Build history of the part. All positions in model axes, mm. Round coordinates to 2 decimals unless told otherwise and drop trailing zeros. Write each loop counter-clockwise with the first axis right and the second up, starting at its lowest first coordinate (ties: lowest second). Pieces come first, ordered by that corner, then holes.
1) Wall check: probe 1 along Y at (x, z) = (-49.5, 1.35); probe 2 along X at (y, z) = (5.5, -0.4); probe 3 along X at (y, z) = (3.75, -1.1). Give the ranges that are in metal, low to high.
2) Saw through at C-C (x = 53). Write the cut outline in (y, z).
3) Saw through at B-B (y = 0). Write the cut outline in (x, z).
4) Saw through at A-A (z = -0.05). Write the cut outline in (x, y).
5) Saw through at D-D (y = -10). Write the cut outline in (x, z).
6) Flat gauge pins, fed straight in: pin 1 (1 mm diameter, centred on y = 9.5, z = -0.5, fed in from -X); pin 2 (1 mm diameter, centred on y = 9, z = 0.5, fed in from -X); pin 3 (1 mm diameter, centred on y = -2, z = -1, fed in from +X). Where does each tip first touch, or does it go through?
Autodesk Inventor part; units mm, degrees
ref_plane "YZ Plane" through (0, 0, 0) normal (1, 0, 0) x (0, 1, 0)
ref_plane "XZ Plane" through (0, 0, 0) normal (0, 1, 0) x (-1, 0, 0)
ref_plane "XY Plane" through (0, 0, 0) normal (0, 0, 1) x (1, 0, 0)
sketch "Esboço1" plane through (0, 0, 0) normal (0, 0, 1) x (1, 0, 0)
  line L0 (-49.5, 0) -> (49.5, 0) construction
  line L1 (-49.5, -15) -> (49.5, -15)
  line L2 (49.5, 15) -> (-49.5, 15)
  arc A0 (-49.5, 15) -> (-49.5, -15) centre (-49.5, 0) ccw
  arc A1 (49.5, -15) -> (49.5, 15) centre (49.5, 0) ccw
  circle A2 centre (-49.5, 0) radius 8
  circle A3 centre (49.5, 0) radius 8
  point P0 (0, 0)
  dimension "d0" = 16
  dimension "d1" = 99
  dimension "d4" = 30
extrude "Extrusão1" add sketch "Esboço1" along normal mid plane 3
sketch "Esboço2" plane through (0, 0, 1.5) normal (0, 0, 1) x (1, 0, 0)
  circle A0 centre (-49.5, 0) radius 8
  circle A1 centre (49.5, 0) radius 8
  line L0 (-49.5, 0) -> (49.5, 0)
  line L1 (0, 0) -> (0, -34.993)
properties part number "Chapa - Aperto fixação"
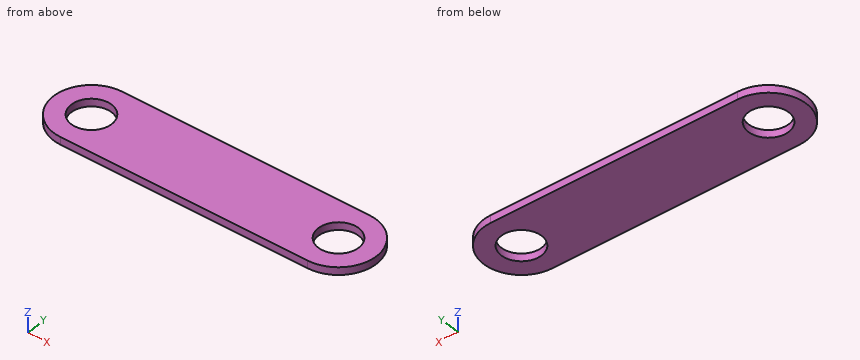
Evaluation:
1. probe 1: y = -15 to -8, 8 to 15
1. probe 2: x = -63.46 to -55.31, -43.69 to 43.69, 55.31 to 63.46
1. probe 3: x = -64.02 to -56.57, -42.43 to 42.43, 56.57 to 64.02
2. outline: (-14.59, -1.5) - (-7.19, -1.5) - (-7.19, 1.5) - (-14.59, 1.5) - close; (7.19, -1.5) - (14.59, -1.5) - (14.59, 1.5) - (7.19, 1.5) - close
3. outline: (-64.5, -1.5) - (-57.5, -1.5) - (-57.5, 1.5) - (-64.5, 1.5) - close; (-41.5, -1.5) - (41.5, -1.5) - (41.5, 1.5) - (-41.5, 1.5) - close; (57.5, -1.5) - (64.5, -1.5) - (64.5, 1.5) - (57.5, 1.5) - close
4. outline: (-49.5, -15) - (49.5, -15) arc R15 ccw to (49.5, 15) - (-49.5, 15) arc R15 ccw to start; hole circle Ø16 at (-49.5, 0); hole circle Ø16 at (49.5, 0)
5. outline: (-60.68, -1.5) - (60.68, -1.5) - (60.68, 1.5) - (-60.68, 1.5) - close
6. pin 1: stops at x = -61.5
6. pin 2: stops at x = -61.86
6. pin 3: stops at x = 64.42
